```python
from build123d import *

# Parameters (mm, degrees)
BOSS_EXTRU_1_DEPTH = 100


with BuildPart() as part:
    # Esquisse1 → Boss.-Extru.1 (new body)
    with BuildSketch(Plane.XY):
        with BuildLine():
            Line((22.500000043, 5.099999967), (22.500000043, 19.499999968))
            ThreePointArc((22.500000043, 19.499999968), (21.621320369, 21.621320326), (19.500000002, 22.499999981))
            Line((19.500000002, 22.499999981), (5.100000002, 22.499999981))
            Line((5.100000002, 22.499999981), (5.100000002, 16.499999976))
            Line((5.100000002, 16.499999976), (10.050000002, 16.499999976))
            Line((10.050000002, 16.499999976), (10.050000002, 12.121320348))
            Line((10.050000002, 12.121320348), (7.378679628, 9.499999975))
            Line((7.378679628, 9.499999975), (0.51961526, 9.499999975))
            Line((0.51961526, 9.499999975), (1.4e-08, 9.199999973))
            Line((1.4e-08, 9.199999973), (-0.519615231, 9.499999975))
            Line((-0.519615231, 9.499999975), (-7.3786796, 9.499999975))
            Line((-7.3786796, 9.499999975), (-10.049999998, 12.121320324))
            Line((-10.049999998, 12.121320324), (-10.049999998, 16.499999952))
            Line((-10.049999998, 16.499999952), (-5.099999998, 16.499999952))
            Line((-5.099999998, 16.499999952), (-5.099999998, 22.499999958))
            Line((-5.099999998, 22.499999958), (-19.499999998, 22.499999958))
            ThreePointArc((-19.499999998, 22.499999958), (-21.621320357, 21.621320284), (-22.500000012, 19.499999917))
            Line((-22.500000012, 19.499999917), (-22.500000012, 5.099999917))
            Line((-22.500000012, 5.099999917), (-16.500000006, 5.099999917))
            Line((-16.500000006, 5.099999917), (-16.500000006, 10.049999917))
            Line((-16.500000006, 10.049999917), (-12.121320378, 10.049999917))
            Line((-12.121320378, 10.049999917), (-9.500000005, 7.378679543))
            Line((-9.500000005, 7.378679543), (-9.500000005, 0.519615174))
            Line((-9.500000005, 0.519615174), (-9.200000003, -7.1e-08))
            Line((-9.200000003, -7.1e-08), (-9.500000005, -0.519615317))
            Line((-9.500000005, -0.519615317), (-9.500000005, -7.378679686))
            Line((-9.500000005, -7.378679686), (-12.121320354, -10.050000083))
            Line((-12.121320354, -10.050000083), (-16.499999982, -10.050000083))
            Line((-16.499999982, -10.050000083), (-16.499999982, -5.100000083))
            Line((-16.499999982, -5.100000083), (-22.499999988, -5.100000083))
            Line((-22.499999988, -5.100000083), (-22.499999988, -19.500000083))
            ThreePointArc((-22.499999988, -19.500000083), (-21.621320314, -21.621320442), (-19.499999947, -22.500000097))
            Line((-19.499999947, -22.500000097), (-5.099999947, -22.500000097))
            Line((-5.099999947, -22.500000097), (-5.099999947, -16.500000091))
            Line((-5.099999947, -16.500000091), (-10.049999947, -16.500000091))
            Line((-10.049999947, -16.500000091), (-10.049999947, -12.121320464))
            Line((-10.049999947, -12.121320464), (-7.378679573, -9.500000091))
            Line((-7.378679573, -9.500000091), (-0.519615204, -9.500000091))
            Line((-0.519615204, -9.500000091), (4.1e-08, -9.200000089))
            Line((4.1e-08, -9.200000089), (0.519615287, -9.500000091))
            Line((0.519615287, -9.500000091), (7.378679655, -9.500000091))
            Line((7.378679655, -9.500000091), (10.050000053, -12.12132044))
            Line((10.050000053, -12.12132044), (10.050000053, -16.500000068))
            Line((10.050000053, -16.500000068), (5.100000053, -16.500000068))
            Line((5.100000053, -16.500000068), (5.100000053, -22.500000073))
            Line((5.100000053, -22.500000073), (19.500000053, -22.500000073))
            ThreePointArc((19.500000053, -22.500000073), (21.621320412, -21.621320399), (22.500000067, -19.500000033))
            Line((22.500000067, -19.500000033), (22.500000067, -5.100000033))
            Line((22.500000067, -5.100000033), (16.500000061, -5.100000033))
            Line((16.500000061, -5.100000033), (16.500000061, -10.050000033))
            Line((16.500000061, -10.050000033), (12.121320433, -10.050000033))
            Line((12.121320433, -10.050000033), (9.50000006, -7.378679659))
            Line((9.50000006, -7.378679659), (9.50000006, -0.51961529))
            Line((9.50000006, -0.51961529), (9.200000058, -4.4e-08))
            Line((9.200000058, -4.4e-08), (9.50000006, 0.519615201))
            Line((9.50000006, 0.519615201), (9.50000006, 7.37867957))
            Line((9.50000006, 7.37867957), (12.12132041, 10.049999967))
            Line((12.12132041, 10.049999967), (16.500000038, 10.049999967))
            Line((16.500000038, 10.049999967), (16.500000038, 5.099999967))
            Line((16.500000038, 5.099999967), (22.500000043, 5.099999967))
        make_face()
        with BuildLine():
            Line((15.855339158, -20.207106708), (20.207106825, -15.855339041))
            ThreePointArc((20.207106825, -15.855339041), (20.4238796, -15.530915671), (20.500000069, -15.148232209))
            Line((20.500000069, -15.148232209), (20.500000069, -11.54999993))
            ThreePointArc((20.500000069, -11.54999993), (19.388228621, -10.101111187), (17.700961947, -10.79999996))
            ThreePointArc((17.700961947, -10.79999996), (17.334936545, -11.166025343), (16.83493656, -11.299999931))
            Line((16.83493656, -11.299999931), (11.800000069, -11.299999931))
            ThreePointArc((11.800000069, -11.299999931), (11.446446677, -11.446446542), (11.300000069, -11.799999935))
            Line((11.300000069, -11.799999935), (11.300000069, -16.834936434))
            ThreePointArc((11.300000069, -16.834936434), (11.166025484, -17.334936416), (10.800000106, -17.700961817))
            ThreePointArc((10.800000106, -17.700961817), (10.101111348, -19.388228497), (11.550000101, -20.499999933))
            Line((11.550000101, -20.499999933), (15.14823238, -20.499999933))
            ThreePointArc((15.14823238, -20.499999933), (15.530915811, -20.423879462), (15.855339158, -20.207106708))
        make_face(mode=Mode.SUBTRACT)
        with BuildLine():
            Line((-20.499999933, -11.550000112), (-20.499999933, -15.148232391))
            ThreePointArc((-20.499999933, -15.148232391), (-20.423879462, -15.530915822), (-20.207106708, -15.855339169))
            Line((-20.207106708, -15.855339169), (-15.855339041, -20.207106836))
            ThreePointArc((-15.855339041, -20.207106836), (-15.530915692, -20.423879587), (-15.14823226, -20.500000055))
            Line((-15.14823226, -20.500000055), (-11.549999982, -20.500000055))
            ThreePointArc((-11.549999982, -20.500000055), (-10.101111238, -19.388228606), (-10.800000011, -17.700961932))
            ThreePointArc((-10.800000011, -17.700961932), (-11.166025359, -17.334936533), (-11.299999931, -16.834936571))
            Line((-11.299999931, -16.834936571), (-11.299999931, -11.80000008))
            ThreePointArc((-11.299999931, -11.80000008), (-11.446446542, -11.446446688), (-11.799999935, -11.30000008))
            Line((-11.799999935, -11.30000008), (-16.834936426, -11.30000008))
            ThreePointArc((-16.834936426, -11.30000008), (-17.334936412, -11.166025497), (-17.700961817, -10.800000117))
            ThreePointArc((-17.700961817, -10.800000117), (-19.388228497, -10.101111359), (-20.499999933, -11.550000112))
        make_face(mode=Mode.SUBTRACT)
        with BuildLine():
            Line((-15.85533915, 20.20710669), (-20.207106817, 15.855339024))
            ThreePointArc((-20.207106817, 15.855339024), (-20.423879568, 15.530915675), (-20.500000035, 15.148232242))
            Line((-20.500000035, 15.148232242), (-20.500000035, 11.549999964))
            ThreePointArc((-20.500000035, 11.549999964), (-19.388228587, 10.101111221), (-17.700961913, 10.799999993))
            ThreePointArc((-17.700961913, 10.799999993), (-17.334936511, 11.166025377), (-16.834936526, 11.299999965))
            Line((-16.834936526, 11.299999965), (-11.800000035, 11.299999965))
            ThreePointArc((-11.800000035, 11.299999965), (-11.446446643, 11.446446576), (-11.300000035, 11.799999969))
            Line((-11.300000035, 11.799999969), (-11.300000035, 16.834936459))
            ThreePointArc((-11.300000035, 16.834936459), (-11.16602545, 17.334936413), (-10.800000097, 17.7009618))
            ThreePointArc((-10.800000097, 17.7009618), (-10.10111134, 19.38822848), (-11.550000093, 20.499999915))
            Line((-11.550000093, 20.499999915), (-15.148232371, 20.499999915))
            ThreePointArc((-15.148232371, 20.499999915), (-15.530915803, 20.423879445), (-15.85533915, 20.20710669))
        make_face(mode=Mode.SUBTRACT)
        with BuildLine():
            Line((-3.600000106, 7.899999961), (-7.399999998, 7.899999961))
            ThreePointArc((-7.399999998, 7.899999961), (-7.753553388, 7.75355335), (-7.899999996, 7.399999959))
            Line((-7.899999996, 7.399999959), (-7.899999996, 3.600000067))
            ThreePointArc((-7.899999996, 3.600000067), (-7.676191867, 3.132581845), (-7.171734284, 3.013870341))
            ThreePointArc((-7.171734284, 3.013870341), (-6.226759165, 2.719151967), (-5.99823974, 1.75602385))
            ThreePointArc((-5.99823974, 1.75602385), (-6.249999979, -2.2e-08), (-5.998239727, -1.756023893))
            ThreePointArc((-5.998239727, -1.756023893), (-6.226759144, -2.719152011), (-7.171734261, -3.013870394))
            ThreePointArc((-7.171734261, -3.013870394), (-7.676191842, -3.132581902), (-7.899999967, -3.600000126))
            Line((-7.899999967, -3.600000126), (-7.899999967, -7.400000018))
            ThreePointArc((-7.899999967, -7.400000018), (-7.753553356, -7.753553408), (-7.399999965, -7.900000016))
            Line((-7.399999965, -7.900000016), (-3.600000073, -7.900000016))
            ThreePointArc((-3.600000073, -7.900000016), (-3.132581851, -7.676191887), (-3.013870347, -7.171734304))
            ThreePointArc((-3.013870347, -7.171734304), (-2.719151972, -6.226759185), (-1.756023856, -5.99823976))
            ThreePointArc((-1.756023856, -5.99823976), (2.8e-08, -6.25), (1.756023909, -5.998239744))
            ThreePointArc((1.756023909, -5.998239744), (2.719152028, -6.226759161), (3.013870411, -7.171734278))
            ThreePointArc((3.013870411, -7.171734278), (3.132581919, -7.676191859), (3.600000143, -7.899999984))
            Line((3.600000143, -7.899999984), (7.400000035, -7.899999984))
            ThreePointArc((7.400000035, -7.899999984), (7.75355342, -7.753553361), (7.900000016, -7.399999965))
            Line((7.900000016, -7.399999965), (7.900000016, -3.600000073))
            ThreePointArc((7.900000016, -3.600000073), (7.676191887, -3.132581851), (7.171734305, -3.013870347))
            ThreePointArc((7.171734305, -3.013870347), (6.226759185, -2.719151972), (5.99823976, -1.756023856))
            ThreePointArc((5.99823976, -1.756023856), (6.25, 2.8e-08), (5.998239744, 1.756023909))
            ThreePointArc((5.998239744, 1.756023909), (6.226759161, 2.719152028), (7.171734278, 3.013870411))
            ThreePointArc((7.171734278, 3.013870411), (7.676191859, 3.132581919), (7.899999984, 3.600000143))
            Line((7.899999984, 3.600000143), (7.899999984, 7.400000035))
            ThreePointArc((7.899999984, 7.400000035), (7.753553347, 7.753553403), (7.399999956, 7.899999985))
            Line((7.399999956, 7.899999985), (3.600000064, 7.899999985))
            ThreePointArc((3.600000064, 7.899999985), (3.132581842, 7.676191856), (3.013870338, 7.171734274))
            ThreePointArc((3.013870338, 7.171734274), (2.719151963, 6.226759154), (1.756023847, 5.998239729))
            ThreePointArc((1.756023847, 5.998239729), (-1.3e-08, 6.249999968), (-1.756023872, 5.998239721))
            ThreePointArc((-1.756023872, 5.998239721), (-2.719151991, 6.226759139), (-3.013870374, 7.171734255))
            ThreePointArc((-3.013870374, 7.171734255), (-3.132581882, 7.676191836), (-3.600000106, 7.899999961))
        make_face(mode=Mode.SUBTRACT)
        with BuildLine():
            Line((11.299999964, 16.83493656), (11.299999964, 11.800000069))
            ThreePointArc((11.299999964, 11.800000069), (11.446446575, 11.446446677), (11.799999969, 11.300000069))
            Line((11.799999969, 11.300000069), (16.834936459, 11.300000069))
            ThreePointArc((16.834936459, 11.300000069), (17.334936446, 11.166025486), (17.700961851, 10.800000106))
            ThreePointArc((17.700961851, 10.800000106), (19.388228531, 10.101111348), (20.499999967, 11.550000101))
            Line((20.499999967, 11.550000101), (20.499999967, 15.14823238))
            ThreePointArc((20.499999967, 15.14823238), (20.423879472, 15.530915844), (20.207106671, 15.855339203))
            Line((20.207106671, 15.855339203), (15.855339024, 20.207106851))
            ThreePointArc((15.855339024, 20.207106851), (15.530915675, 20.423879602), (15.148232242, 20.500000069))
            Line((15.148232242, 20.500000069), (11.549999964, 20.500000069))
            ThreePointArc((11.549999964, 20.500000069), (10.10111122, 19.388228621), (10.799999993, 17.700961947))
            ThreePointArc((10.799999993, 17.700961947), (11.166025377, 17.334936545), (11.299999964, 16.83493656))
        make_face(mode=Mode.SUBTRACT)
    extrude(amount=BOSS_EXTRU_1_DEPTH)


solid = part.part
```
Could you check a few things on this model? Use its own coordinates, in mm. A direction names the side the tool comes from. Round coordinates to 2 decimals unless told otherwise and drop trailing zeros. Write each question's results on one line, items separated by ' | '. Start each with the question number.
1. I'm going to push a flat-ended pin straight in: pin 1 Ø3.5 at (x, z) = (3, 73) entering from +Y. Where does the tip first touch, or does it pass through?
2. Imagine slicing it at A-A on z = 73.5. Count the separate pieces of the cut face and the enclosed holes in it, and give its area (3 significant figures).
3. I need wall thicknesses on L1, parallel to X at y = 15, z = 91.5; L2, parallel to Y at x = -2, z = 83.5; L3, parallel to Y at x = -9, z = 19. Which ranges of each line are inside material? Lowest first, please. Write a range as from..to.
4. On a 3-axis mill with a long thin cutter (end or side, diameter ignored), from which of +Z, -Z, +X, -X, +Y, -Y can I reach the whole of each face in a straight line? I mean faces 1 (the face through (-10.094, 19.362, 49.3)), 2 (the face through (-5.1, -20, 49)). Say none if no direction works.
5. Thinking about a two-plate mould opening in X: for faces 3 (the face through (16.5, -8, 49)), 4 (the face through (2, 7, 0)), which applies, +X half, -X half, draft (parallel to the pull), parting line (faces both ways), or undercut?
Result sheet:
1) pin 1: stops at y = 9.5
2) separate pieces: 1 | enclosed holes: 5 | area: 718 mm^2
3) L1: x = -22.5..-20.5, -11.3..-10.05, 10.05..11.3, 20.5..22.5 | L2: y = -9.5..-5.96, 5.96..9.5 | L3: y = -22.5..-16.5, -11.09..11.09, 16.5..22.5
4) face 1: +Z, -Z | face 2: +Z, -Z, -Y
5) face 3: undercut | face 4: draft
